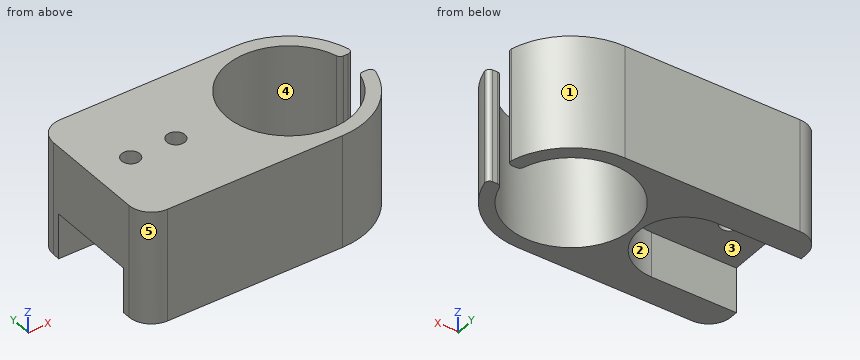
from build123d import *

# Parameters (mm, degrees)
ESQUISSE1_R             = 2
BOSS_EXTRU_1_DEPTH      = 25
CONG_1_R                = 5
CONG_2_R                = 1
ENL_V_MAT_EXTRU_1_DEPTH = 10


with BuildPart() as part:
    # Esquisse1 → Boss.-Extru.1 (new body)
    with BuildSketch(Plane.XY):
        with BuildLine():
            Line((13.4187369, 3), (16.479153498, 3))
            ThreePointArc((16.479153498, 3), (10.731088016, 12.861036117), (0, 16.75))
            Line((0, 16.75), (-43.75, 16.75))
            Line((-43.75, 16.75), (-43.75, -16.75))
            Line((-43.75, -16.75), (0, -16.75))
            ThreePointArc((0, -16.75), (10.731088016, -12.861036117), (16.479153498, -3))
            Line((16.479153498, -3), (13.4187369, -3))
            ThreePointArc((13.4187369, -3), (-13.75, 0), (13.4187369, 3))
        make_face()
        with Locations((-35, 0)):
            Circle(ESQUISSE1_R, mode=Mode.SUBTRACT)
        with Locations((-25, 0)):
            Circle(ESQUISSE1_R, mode=Mode.SUBTRACT)
    extrude(amount=BOSS_EXTRU_1_DEPTH)

    # Congé1
    cong_1_edges = [part.edges().sort_by_distance(p)[0] for p in [
        (-43.75, -16.75, 12.5),
        (-43.75, 16.75, 12.5),
    ]]
    fillet(cong_1_edges, radius=CONG_1_R)

    # Congé2
    cong_2_edges = [part.edges().sort_by_distance(p)[0] for p in [
        (13.4187369, -3, 12.5),
        (16.479153498, -3, 12.5),
        (16.479153498, 3, 12.5),
        (13.4187369, 3, 12.5),
    ]]
    fillet(cong_2_edges, radius=CONG_2_R)

    # Esquisse2 → Enlèv. mat.-Extru.1 (cut)
    with BuildSketch(Plane(origin=(0, 0, 0), x_dir=(-1, 0, 0), z_dir=(0, 0, -1))):
        with BuildLine():
            Line((43.75, 10.1), (25, 10.1))
            ThreePointArc((25, 10.1), (14.9, 0), (25, -10.1))
            Line((25, -10.1), (43.75, -10.1))
            Line((43.75, -10.1), (43.75, 10.1))
        make_face()
    extrude(amount=-ENL_V_MAT_EXTRU_1_DEPTH, mode=Mode.SUBTRACT)


solid = part.part
Build history of the part. All positions in model axes, mm. Face numbers are marked on the shaded views. A direction names the side the tool comes from. Coordinates: 2 decimals unless noted, no trailing zeros. Write each loop counter-clockwise with the first axis right and the second up, starting at its lowest first coordinate (ties: lowest second). Pieces come first, ordered by that corner, then holes. Notation, with made-up numbers: (-38.75, 36) -> (2.25, 36) arc R20 ccw to (2.25, 51) -> close; hole circle Ø11 at (20.25, 23). An arc over 180 degrees is marked (long way). Use CSV: the item, a comma, the result in double quotes. Start each with the question number.
Q1. Cut at B-B, the plane z = 13. List the corners of the cut face in (x, y).
Q2. Cut at D-D, the plane z = 7. List the corners of the cut face in (x, y).
Q3. Drill centre lines: probe 1 along X at (y, z) = (0, 17); probe 2 along Y at (x, z) = (-35, 20.5); probe 3 along Y at (x, z) = (-27, 4.25). Where is each one in solid material? Low to high.
Q4. Cut at A-A, the plane y = 0. List the corners of the cut face in (x, z), then the cut area to 4 significant figures.
Q5. Flat gauge pins, fed straight in: pin 1 Ø4.5 at (x, y) = (-35, 0) entering from -Z; pin 2 Ø0.8 at (x, z) = (14.5, 7.5) entering from -Y; pin 3 Ø6 at (y, z) = (10, 12) entering from +X. Where does each tip first touch, or does it go through?
Q6. Pull direction X, two halves, no side cores. Call the marked faces 3, 4 and 5: released by +X, released by -X, zero draft, split by the parting line, or undercut.
Q7. Cut at C-C, the plane x = -35. List the corners of the cut face in (y, z), then the cut area to 4 significant figures.
Q8. 3-axis set-ups, long thin cutter, end or side, ignore diameter. For the marked faces 1 and 2: which of +Z, -Z, +X, -X, +Y, -Y reach the whole face in a straight line?
Checked values:
1,outline,"(-43.75, -11.75) arc R5 ccw to (-38.75, -16.75) -> (0, -16.75) arc R16.75 ccw to (16.2, -4.25) arc R1 ccw to (15.23, -3) -> (14.2, -3) arc R1 ccw to (13.23, -3.73) arc R13.75 cw (long way) to (13.23, 3.73) arc R1 ccw to (14.2, 3) -> (15.23, 3) arc R1 ccw to (16.2, 4.25) arc R16.75 ccw to (0, 16.75) -> (-38.75, 16.75) arc R5 ccw to (-43.75, 11.75) -> close; hole circle Ø4 at (-35, 0); hole circle Ø4 at (-25, 0)"
2,outline,"(-43.75, -11.75) arc R5 ccw to (-38.75, -16.75) -> (0, -16.75) arc R16.75 ccw to (16.2, -4.25) arc R1 ccw to (15.23, -3) -> (14.2, -3) arc R1 ccw to (13.23, -3.73) arc R13.75 cw (long way) to (13.23, 3.73) arc R1 ccw to (14.2, 3) -> (15.23, 3) arc R1 ccw to (16.2, 4.25) arc R16.75 ccw to (0, 16.75) -> (-38.75, 16.75) arc R5 ccw to (-43.75, 11.75) -> (-43.75, 10.1) -> (-25, 10.1) arc R10.1 cw to (-25, -10.1) -> (-43.75, -10.1) -> close"
3,probe 1,"x = -43.75 to -37, -33 to -27, -23 to -13.75"
3,probe 2,"y = -16.75 to -2, 2 to 16.75"
3,probe 3,"y = -16.75 to -10.1, 10.1 to 16.75"
4,outline,"(-43.75, 10) -> (-37, 10) -> (-37, 25) -> (-43.75, 25) -> close; (-33, 10) -> (-27, 10) -> (-27, 25) -> (-33, 25) -> close; (-23, 10) -> (-14.9, 10) -> (-14.9, 0) -> (-13.75, 0) -> (-13.75, 25) -> (-23, 25) -> close"
4,area,"341.5 mm²"
5,pin 1,"stops at z = 10"
5,pin 2,"stops at y = -9.04"
5,pin 3,"stops at x = 15.22"
6,face 3,"zero draft"
6,face 4,"undercut"
6,face 5,"released by -X"
7,outline,"(-16.75, 0) -> (-10.1, 0) -> (-10.1, 10) -> (-2, 10) -> (-2, 25) -> (-16.75, 25) -> close; (2, 10) -> (10.1, 10) -> (10.1, 0) -> (16.75, 0) -> (16.75, 25) -> (2, 25) -> close"
7,area,"575.5 mm²"
8,face 1,"+Z, -Z, +X, +Y"
8,face 2,"-Z, -X"
